Verification items for this drawing (mm, ordinates from the low corner). A direction names the side the tool comes from. Coordinates: 2 decimals unless noted, no trailing zeros. Loops run counter-clockwise (first coordinate to the right, second up) from the corner with the lowest first, then second, coordinate; pieces in that order, holes last. Notation, with made-up numbers: (-35.75, 69.25) -> (-29.75, 69.25) arc R6 cw to (-29.75, 80.25) -> close; hole circle Ø5 at (-37, 71.5). An arc over 180 degrees is marked (long way). Write item = value, one per line.
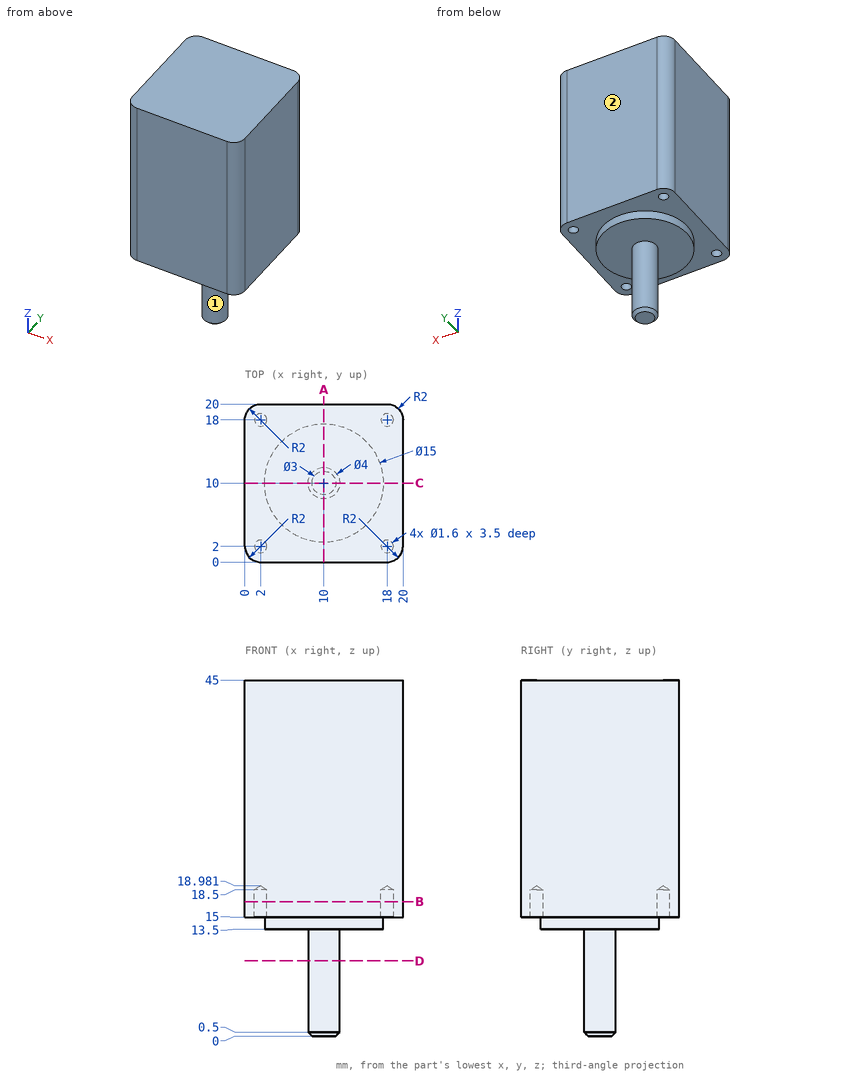
1) Sectioned sample at A-A, the plane x = 10. Record the cut outline in (y, z), plus the area to 3 significant figures.
Ans:
outline = (0, 15) -> (2.5, 15) -> (2.5, 13.5) -> (8, 13.5) -> (8, 0.5) -> (8.5, 0) -> (11.5, 0) -> (12, 0.5) -> (12, 13.5) -> (17.5, 13.5) -> (17.5, 15) -> (20, 15) -> (20, 45) -> (0, 45) -> close
area = 676 mm2
2) Material ranges on line 1 (Y direction, x = 18, z = 15.7); line 2 (Z direction, x = 17, y = 9.5), recorded low to high.
Ans:
line_1 = 0 to 1.2, 2.8 to 17.2, 18.8 to 20
line_2 = 13.5 to 45
3) Sectioned sample at B-B, the plane z = 17. Record the cut outline in (x, y).
Ans:
outline = (0, 2) arc R2 ccw to (2, 0) -> (18, 0) arc R2 ccw to (20, 2) -> (20, 18) arc R2 ccw to (18, 20) -> (2, 20) arc R2 ccw to (0, 18) -> close; hole circle Ø1.6 at (2, 2); hole circle Ø1.6 at (2, 18); hole circle Ø1.6 at (18, 2); hole circle Ø1.6 at (18, 18)
4) Tool access check on the marked faces 1 and 2. Record the directions out of +Z, -Z, +X, -X, +Y, -Y that give a thin tool (end or side, any length) a straight path to the whole face; none if there is none.
Ans:
face_1 = -Z
face_2 = +Z, -Z, +X, -X, +Y
5) Depth check by flat-ended pin: pin 1 Ø12 at (x, z) = (4.5, 6) entering from -Y; pin 2 Ø1.4 at (x, y) = (18, 2) entering from -Z; pin 3 Ø2 at (x, y) = (2, 2) entering from -Z; pin 4 Ø4 at (y, z) = (5.5, 9) entering from -X. Enter the tip coordinate at first touch or a pass-through.
Ans:
pin_1 = 8
pin_2 = 18.56
pin_3 = 15
pin_4 = through
6) Sectioned sample at D-D, the plane z = 9.5. Record the cut outline in (x, y).
Ans:
outline = circle Ø4 at (10, 10)
